from build123d import *

# Parameters (mm, degrees)
F1_DEPTH = 25.4
F2_R     = 20.5214520654
F3_DEPTH = 25.4
F4_R     = 7.62


# Not quite as in the source:
# - the program builds the solid bodies; features that only make, move or delete a surface that nothing else refers to are left out


with BuildPart() as f1:
    # F0 (on Top) → F1 (new body)
    with BuildSketch(Plane.XY):
        Polygon((65.0288537145, 60.4610182345), (-57.2496131063, 60.4610182345), (-53.2582976497, -16.6874233163), (43.3438569307, -37.969596684), align=None)
    extrude(amount=F1_DEPTH)

    # F2 (on face) → F3 (join)
    with BuildSketch(Plane.XY.offset(25.4)):
        with Locations((-13.8034075499, 21.8867974591)):
            Circle(F2_R)
    extrude(amount=F3_DEPTH)

    # F4
    f4_edges = [f1.edges().sort_by_distance(p)[0] for p in [
        (54.186355, 11.245711, 25.4),
        (-4.95722, -27.32851, 25.4),
        (3.88962, 60.461018, 25.4),
        (-55.253955, 21.886797, 25.4),
        (-34.32486, 21.886797, 25.4),
        (43.343857, -37.969597, 12.7),
        (-4.95722, -27.32851, 0),
    ]]
    fillet(f4_edges, radius=F4_R)


solid = f1.part
Geometry check sheet. Reference: the model listing, model coordinates, mm. A direction names the side the tool comes from. Round coordinates to 2 decimals unless told otherwise and drop trailing zeros. Order: outer loops, then holes, each group sorted by start corner. A loop starts at its lowest first (then second) coordinate and runs counter-clockwise, first axis right, second up. Notation, with made-up numbers: M -32.75,65.25 L -7.75,65.25 A31 ccw -7.75,103.25 Z; hole C 74,74.5 d3. An arc over 180 degrees is marked long. Answer in a Markdown table with one row per item.
(1) Tool access check on faces 1 (the face through (54.866, 14.33, 8.766)), 2 (the face through (-30.09, 9.4, 41.79)). Record the directions out of +Z, -Z, +X, -X, +Y, -Y that give a thin tool (end or side, any length) a straight path to the whole face; none if there is none.
Responses:
| item | result |
|---|---|
| face 1 | +Z, -Z, +X, -Y |
| face 2 | +Z |
(2) Go/stop test with flat-tipped pins: P1, Ø4, axis at x = 42.5, z = 29, coming from the -Y side; P2, Ø5, axis at x = 43, z = 24, coming from the +Y side; P3, Ø3, axis at x = -4.5, z = 21.5, coming from the -Y side; P4, Ø1, axis at y = 50, z = 21.5, coming from the -X side. Record where each tip stops, or that it passes through.
Responses:
| item | result |
|---|---|
| P1 | passes through |
| P2 | stops at y = 59.49 |
| P3 | stops at y = -27.19 |
| P4 | stops at x = -56 |
(3) Sectioned sample at C-C, the plane z = 42. Record the cut outline in (x, y), and give its area (3 significant figures).
Responses:
| item | result |
|---|---|
| outline | C -13.8,21.89 d41.04 |
| area | 1,320 mm² |
(4) Sectioned sample at A-A, the plane z = 16. Record the cut outline in (x, y).
Responses:
| item | result |
|---|---|
| outline | M -57.25,60.46 L -53.26,-16.69 L 35.9,-36.33 A7.62 ccw 44.98,-30.53 L 65.03,60.46 Z |
(5) Scan lines: probe 1 along Z at (x, y) = (6, -5); probe 2 along Y at (x, z) = (27.5, 23); probe 3 along X at (y, z) = (-10, 18). Record each from-to range of solid material in increasing order. Write a range as from..to.
Responses:
| item | result |
|---|---|
| probe 1 | z = 0..25.4 |
| probe 2 | y = -32.36..58.39 |
| probe 3 | x = -53.6..49.5 |
(6) Sectioned sample at B-B, the plane z = 29.5. Record the cut outline in (x, y), and give its area (3 significant figures).
Responses:
| item | result |
|---|---|
| outline | C -13.8,21.89 d42.77 |
| area | 1,440 mm² |
